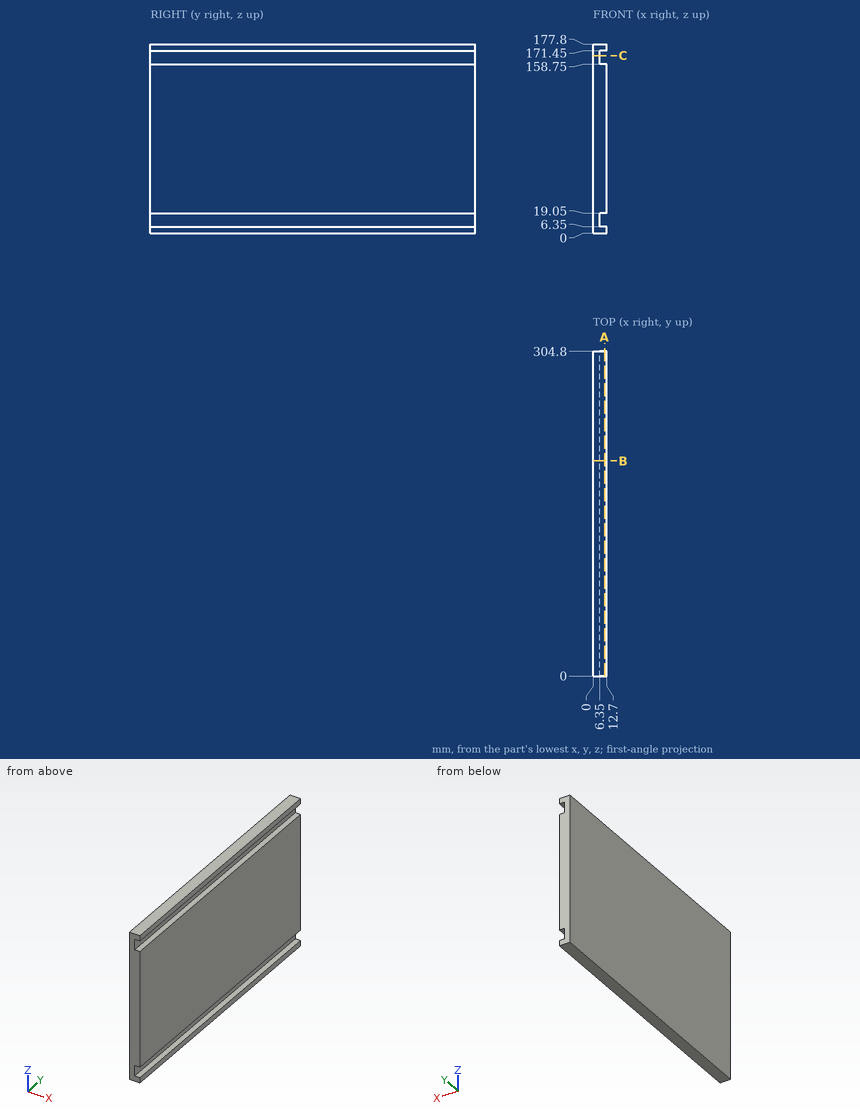
Job drawing, mm, ordinate dimensions from the low corner. One solid piece. Coordinates: 2 decimals unless noted, no trailing zeros. Loops run counter-clockwise (first coordinate to the right, second up) from the corner with the lowest first, then second, coordinate; pieces in that order, holes last. Notation, with made-up numbers: (43.5, 32) - (77.5, 32) arc R24 cw to (77.5, 60) - close; hole circle Ø5 at (4, -10.5). An arc over 180 degrees is marked (long way). Answer as a JSON object with one key per item and string values. Group by question number.
(1) Cut at B-B (y = 202). Give the cut face in (x, z).
(2) Probe line 1 along Z through (x, y) = (10, 28); line 2 along X through (y, z) = (178.5, 15). List the from-to ranges inside material, lowest first.
(3) Cut at A-A (x = 10.75). Give the cut face in (y, z), then the cut area to 3 significant figures.
(4) Cut at C-C (z = 167). Give the cut face in (x, y).
(5) Flat gauge pins, fed straight in: pin 1 (6 mm diameter, centred on y = 123.5, z = 68.5, fed in from -X); pin 2 (4 mm diameter, centred on y = 135, z = 164, fed in from +X). Where does each tip first touch, or does it go through?
Geometry says:
{
 "1": {"outline": "(0, 0) - (12.7, 0) - (12.7, 6.35) - (6.35, 6.35) - (6.35, 19.05) - (12.7, 19.05) - (12.7, 158.75) - (6.35, 158.75) - (6.35, 171.45) - (12.7, 171.45) - (12.7, 177.8) - (0, 177.8) - close"},
 "2": {"line 1": "z = 0 to 6.35, 19.05 to 158.75, 171.45 to 177.8", "line 2": "x = 0 to 6.35"},
 "3": {"outline": "(0, 0) - (304.8, 0) - (304.8, 6.35) - (0, 6.35) - close; (0, 19.05) - (304.8, 19.05) - (304.8, 158.75) - (0, 158.75) - close; (0, 171.45) - (304.8, 171.45) - (304.8, 177.8) - (0, 177.8) - close", "area": "46,500 mm^2"},
 "4": {"outline": "(0, 0) - (6.35, 0) - (6.35, 304.8) - (0, 304.8) - close"},
 "5": {"pin 1": "stops at x = 0", "pin 2": "stops at x = 6.35"}
}
